Source: CAD feature listing. Evaluate the final solid. Frame: model axes, mm. Give positions to 0.01 mm unless a question says otherwise; leave off trailing zeros. Order: outer loops, then holes, each group sorted by start corner. A loop starts at its lowest first (then second) coordinate and runs counter-clockwise, first axis right, second up.
1) Section B-B, the plane y = -11.5. Return loops of the section in (x, z), plus the area to 3 significant figures.
2) Draft query along Y for faces 1 (the face through (1, -15, 0)), 2 (the face through (-16.366, -0.5, 5.1)), 3 (the face through (16.513, -0.219, 4.93)). Return one class per face: released by +Y, released by -Y, zero draft, split by the parting line, or undercut.
3) Section C-C, the plane x = -7.5. Return loops of the section in (y, z), plus the area to 3 significant figures.
4) First-contact query: P1, Ø1.5, axis at x = 7, z = 7, coming from the +Y side; P2, Ø1.5, axis at x = -12, z = 7.5, coming from the +Y side; P3, Ø1, axis at y = -7.5, z = 3.5, coming from the -X side. Flat tips, straight axial feed; report the tip coordinate or a pass-through.
5) Material intervals for line 1 (Y direction, x = 0, z = 6); line 2 (X direction, y = -8.5, z = 4.75); line 3 (X direction, y = 5.5, z = 1.25), sorted ascending.
6) Section A-A, the plane z = 8. Return loops of the section in (x, y).
```python
from build123d import *

# Parameters (mm, degrees)
SKETCH1_R           = 16.514885265
SKETCH1_R_2         = 14.17
BOSS_EXTRUDE1_DEPTH = 10
SKETCH2_W           = 1.74827772
SKETCH2_H           = 14.423291192
CUT_EXTRUDE1_DEPTH  = 1
SKETCH3_W           = 1.31818545
SKETCH3_H           = 5.3419597
CUT_EXTRUDE2_DEPTH  = 0.01


with BuildPart() as part:
    # Sketch1 → Boss-Extrude1 (new body)
    with BuildSketch(Plane.XY):
        Circle(SKETCH1_R)
        Circle(SKETCH1_R_2, mode=Mode.SUBTRACT)
    extrude(amount=BOSS_EXTRUDE1_DEPTH)

    # Sketch2 → Cut-Extrude1 (cut)
    with BuildSketch(Plane(origin=(0, 0, 0), x_dir=(1, 0, 0), z_dir=(0, 1, 0))):
        with Locations((-17.239960851, -5.63132251)):
            Rectangle(SKETCH2_W, SKETCH2_H)
    extrude(amount=-CUT_EXTRUDE1_DEPTH, mode=Mode.SUBTRACT)

    # Sketch3 → Cut-Extrude2 (cut)
    with BuildSketch(Plane.XY):
        with Locations((0.974918477, 15.020333746)):
            Rectangle(SKETCH3_W, SKETCH3_H)
    extrude(amount=CUT_EXTRUDE2_DEPTH, mode=Mode.SUBTRACT)


solid = part.part
```
From the geometry:
1. outline: (-11.85, 0) - (-8.28, 0) - (-8.28, 10) - (-11.85, 10) - close; (8.28, 0) - (11.85, 0) - (11.85, 10) - (8.28, 10) - close
1. area: 71.5 mm2
2. face 1: zero draft
2. face 2: undercut
2. face 3: split by the parting line
3. outline: (-14.71, 0) - (-12.02, 0) - (-12.02, 10) - (-14.71, 10) - close; (12.02, 0) - (14.71, 0) - (14.71, 10) - (12.02, 10) - close
3. area: 53.8 mm2
4. P1: stops at y = 15.29
4. P2: stops at y = 12.09
4. P3: stops at x = -14.96
5. line 1: y = -16.51 to -14.17, 14.17 to 16.51
5. line 2: x = -14.16 to -11.34, 11.34 to 14.16
5. line 3: x = -15.57 to -13.06, 13.06 to 15.57
6. outline: (-16.51, 0) - (-16.37, 0) - (-16.37, -1) - (-16.48, -1) arc R16.51 ccw (long way) to start; hole circle Ø28.34 at (0, 0)
